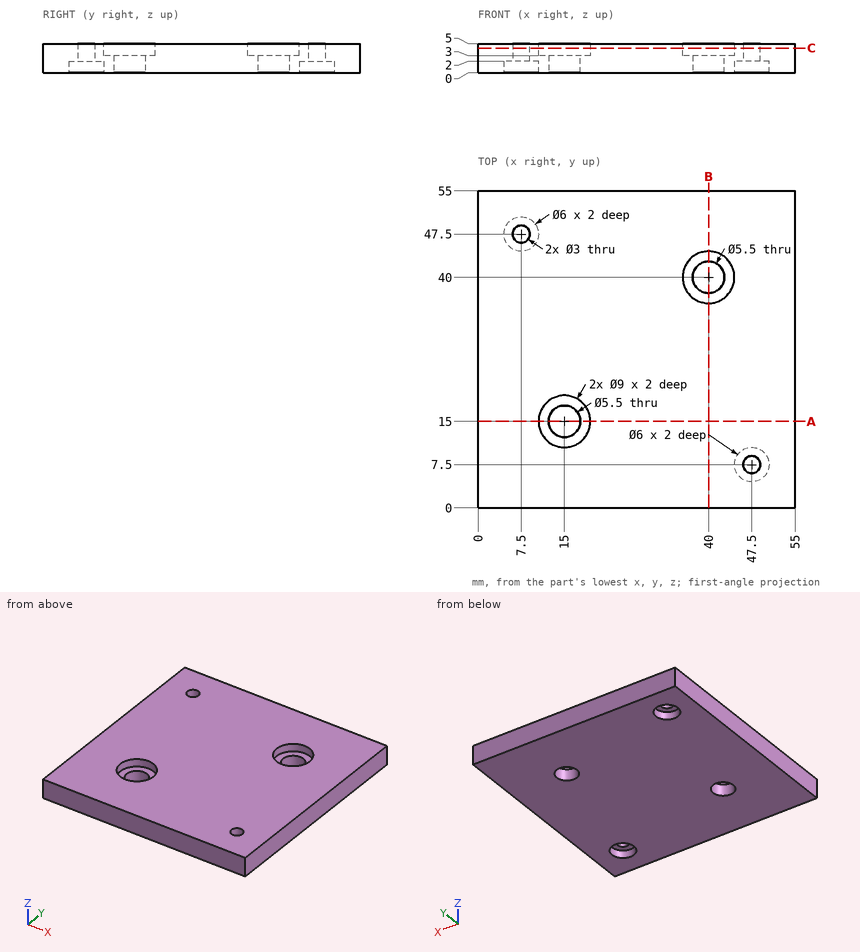
The figure shows three views and two pictorial views of one solid part (mm, origin at its lowest corner). Answer the questions. Give positions to 0.01 mm unless a question says otherwise; leave off trailing zeros. Write each loop counter-clockwise with the first axis right and the second up, starting at its lowest first coordinate (ties: lowest second). Pieces come first, ordered by that corner, then holes. Notation, with made-up numbers: M 66,70.25 L 88,70.25 A31 ccw 88,99.25 Z; hole C 36,-6 d1. An arc over 180 degrees is marked long. Write each question's results on one line, items separated by ' | '.
Q1. Consider L1, parallel to Y at x = 47.5, z = 2.7; L2, parallel to X at y = 15, z = 2; L3, parallel to Z at x = 17, y = 13. Determine where each line is inside the solid, lowest interval first. Write a range as from..to.
Output values:
L1: 0..6, 9..55 | L2: 0..12.25, 17.75..55 | L3: 0..3
Q2. Section B-B, the plane x = 40 is taken. Write down the section's boundary in (y, z).
Output values:
outline: M 0,0 L 37.25,0 L 37.25,3 L 35.5,3 L 35.5,5 L 0,5 Z; M 42.75,0 L 55,0 L 55,5 L 44.5,5 L 44.5,3 L 42.75,3 Z
Q3. Section A-A, the plane y = 15 is taken. Write down the section's boundary in (x, z).
Output values:
outline: M 0,0 L 12.25,0 L 12.25,3 L 10.5,3 L 10.5,5 L 0,5 Z; M 17.75,0 L 55,0 L 55,5 L 19.5,5 L 19.5,3 L 17.75,3 Z
Q4. Flat-ended cylindrical pins translate along their axes: P1, Ø5, axis at x = 7.5, y = 47.5, coming from the -Z side; P2, Ø7, axis at x = 40, y = 40, coming from the +Z side. Find the tip coordinate at first contact, or state that the pin passes through.
Output values:
P1: z = 2 | P2: z = 3
Q5. Section C-C, the plane z = 4.3 is taken. Write down the section's boundary in (x, y).
Output values:
outline: M 0,0 L 55,0 L 55,55 L 0,55 Z; hole C 7.5,47.5 d3; hole C 15,15 d9; hole C 40,40 d9; hole C 47.5,7.5 d3
